Input: part model. Units: mm. Frame: model coordinates. Face numbers are marked on the shaded views. A direction names the side the tool comes from. Give positions to 0.01 mm unless a question says otherwise; leave off trailing zeros. Order: outer loops, then holes, each group sorted by start corner. A loop starts at its lowest first (then second) coordinate and runs counter-clockwise, first axis right, second up. Notation, with made-up numbers: (-5, 24) - (8, 24) arc R21 ccw to (8, 29) - close; hole circle Ø3 at (8, 16). An arc over 180 degrees is marked (long way). Answer in a Markdown table with one row per item. Add a question column.
1. Section query C-C on z = 1.75. Return loops of the section in (x, y), and give its area (3 significant figures).
2. Access query for the marked faces 4, 5, 6, 7 and 8. Directions: +Z, -Z, +X, -X, +Y, -Y. A direction counts if a zero-diameter tool reaches every point of the face in a straight line with its end or side. Return the directions, or none.
3. Ray query, line 1 (X direction, y = 27, z = 1.5); line 2 (Y direction, x = -1.5, z = 0); line 3 (Z direction, x = -10.5, y = 8). Return the intervals inside material, ascending. Write a range as [from, to].
4. Section query D-D on x = -16. Return loops of the section in (y, z).
5. Mould query, pull axis X, two halves, no side actions, for the marked faces 1, 2 and 3. Classes: released by +X, released by -X, zero draft, split by the parting line, or undercut.
6. Section query B-B on x = -2.5. Return loops of the section in (y, z), and give its area (3 significant figures).
7. Contact query for flat-ended pins moving along their axis: pin 1 (6.5 mm diameter, centred on y = 19.5, z = 3, fed in from +X); pin 2 (1.5 mm diameter, centred on x = 7.5, y = 13, fed in from +Z); pin 3 (4 mm diameter, centred on x = -6.5, y = 9, fed in from -Z). Output: stop coordinate, or through.
8. Section query A-A on y = 17.5. Return loops of the section in (x, z).
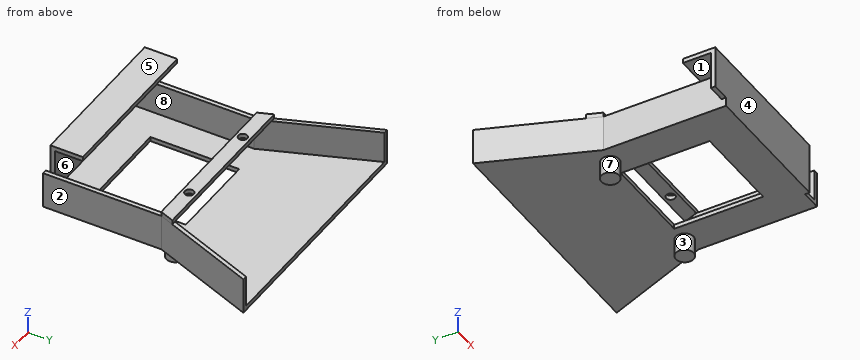
```python
from build123d import *

# Parameters (mm, degrees)
F0_W      = 16.1925
F0_H      = 15.875
F1_DEPTH  = 0.3175
F3_DEPTH  = 5.715
F5_DEPTH  = 0.79375
F6_R      = 0.79375
F7_DEPTH  = 0.79375
F8_DEPTH  = 0.3175
F9_W      = 1.5875
F9_H      = 0.635
F10_DEPTH = 1.5875
F11_DEPTH = 0.3175
F12_W     = 1.5875
F12_H     = 1.5875
F13_DEPTH = 0.79375
F14_DEPTH = 0.15875
F15_R     = 0.5
F16_DEPTH = 25.4
F17_R     = 1.5875
F18_DEPTH = 3.175
F19_DEPTH = 1.5875
F20_DEPTH = 12.7
F21_R     = 0.5
F22_DEPTH = 25.30475
F23_W     = 1.5875
F23_H     = 1.5875
F24_DEPTH = 3.27025
F25_W     = 28.575
F25_H     = 0.79375
F26_DEPTH = 7.62
F27_DEPTH = 0.79375
F28_DEPTH = 0.79375
F29_DEPTH = 0.79375
F30_DEPTH = 25.4
F31_W     = 28.575
F31_H     = 0.79375
F32_DEPTH = 4.998339


with BuildPart() as f1:
    # F0 (on Top) → F1 (new body)
    with BuildSketch(Plane.XY):
        Polygon((-25.671613648, 46.3675076752), (-18.369113648, 27.4050211887), (-18.369113648, 7.0850211887), (10.523386352, 7.0850211887), (10.523386352, 27.4050211887), (17.825886352, 46.3675076752), align=None)
        with Locations((-3.922863648, 20.1025211887)):
            Rectangle(F0_W, F0_H, mode=Mode.SUBTRACT)
    extrude(amount=F1_DEPTH)

    # F2 (on face) → F3 (join)
    with BuildSketch(Plane.XY.offset(0.3175)):
        Polygon((17.825886352, 46.3675076752), (17.032136352, 46.3675076752), (9.729636352, 27.4050211887), (9.729636352, 7.0850211887), (10.523386352, 7.0850211887), (10.523386352, 27.4050211887), align=None)
        Polygon((-24.877863648, 46.3675076752), (-25.671613648, 46.3675076752), (-18.369113648, 27.4050211887), (-18.369113648, 7.0850211887), (-17.575363648, 7.0850211887), (-17.575363648, 27.4050211887), align=None)
    extrude(amount=F3_DEPTH)

    # F4 (on face) → F5 (join)
    with BuildSketch(Plane.XY.offset(6.0325)):
        Polygon((-19.3472738705, 29.9450211887), (-18.369113648, 27.4050211887), (10.523386352, 27.4050211887), (11.5015465745, 29.9450211887), align=None)
    extrude(amount=F5_DEPTH)

    # F6 (on face) → F7 (cut)
    with BuildSketch(Plane.XY.offset(6.82625)):
        with Locations((-12.019113648, 28.6750211887)):
            Circle(F6_R)
        with Locations((4.173386352, 28.6750211887)):
            Circle(F6_R)
    extrude(amount=-F7_DEPTH, mode=Mode.SUBTRACT)

    # F8 (add): a face of the model
    f8_faces = [f1.faces().sort_by_distance(p)[0] for p in [
        (-3.922863648, 30.216271867, 0),
    ]]
    extrude(f8_faces, amount=F8_DEPTH)

    # F9 (on face) → F10 (join)
    with BuildSketch(Plane.XZ.offset(-7.0850211887)):
        Polygon((-17.575363648, 0.3175), (-18.369113648, 0.3175), (-18.369113648, -0.3175), (-16.781613648, -0.3175), (-16.781613648, 0.3175), align=None)
        with Locations((-14.400363648, 0)):
            Rectangle(F9_W, F9_H)
        with Locations((1.379386352, 0)):
            Rectangle(F9_W, F9_H)
        with Locations((4.554386352, 0)):
            Rectangle(F9_W, F9_H)
    extrude(amount=F10_DEPTH)

    # F11 (add): a face of the model
    f11_faces = [f1.faces().sort_by_distance(p)[0] for p in [
        (-3.9482759262, 29.9813117116, -0.3175),
    ]]
    extrude(f11_faces, amount=F11_DEPTH)

    # F12 (on face) → F13 (join)
    with BuildSketch(Plane.XY.offset(0.3175)):
        with Locations((-17.575363648, 6.2912711887)):
            Rectangle(F12_W, F12_H)
        with Locations((-14.400363648, 6.2912711887)):
            Rectangle(F12_W, F12_H)
        with Locations((1.379386352, 6.2912711887)):
            Rectangle(F12_W, F12_H)
        with Locations((4.554386352, 6.2912711887)):
            Rectangle(F12_W, F12_H)
    extrude(amount=F13_DEPTH)

    # F14 (cut): a face of the model
    f14_faces = [f1.faces().sort_by_distance(p)[0] for p in [
        (-3.9482759262, 29.9813117116, -0.635),
    ]]
    extrude(f14_faces, amount=-F14_DEPTH, mode=Mode.SUBTRACT)

    # F15 (on face) → F16 (cut)
    with BuildSketch(Plane(origin=(-18.369113648, 0, 0), x_dir=(0, -1, 0), z_dir=(-1, 0, 0))):
        with Locations((-6.2912711887, 0.3175)):
            Circle(F15_R)
    extrude(amount=-F16_DEPTH, mode=Mode.SUBTRACT)

    # F17 (on face) → F18 (join)
    with BuildSketch(Plane(origin=(0, 0, -0.47625), x_dir=(1, 0, 0), z_dir=(0, 0, -1))):
        with Locations((-15.194113648, -28.0400211887)):
            Circle(F17_R)
        with Locations((7.348386352, -28.0400211887)):
            Circle(F17_R)
    extrude(amount=F18_DEPTH)

    # F19 (add): faces of the model
    f19_faces = [f1.faces().sort_by_distance(p)[0] for p in [
        (5.348136352, 7.0625705484, -0.079375),
        (2.173136352, 7.0625705484, -0.079375),
        (-16.781613648, 7.0625705484, -0.079375),
        (-13.606613648, 7.0625705484, -0.079375),
    ]]
    extrude(f19_faces, amount=F19_DEPTH)

    # F20 (add): a face of the model
    f20_faces = [f1.faces().sort_by_distance(p)[0] for p in [
        (-12.019113648, 6.2912711887, -0.4537993597),
    ]]
    extrude(f20_faces, amount=F20_DEPTH)

    # F21 (on face) → F22 (join)
    with BuildSketch(Plane.YZ.offset(6.935636352)):
        with Locations((6.2912711887, 0.3175)):
            Circle(F21_R)
    extrude(amount=-F22_DEPTH)

    # F23 (on face) → F24 (join)
    with BuildSketch(Plane(origin=(-18.369113648, 0, 0), x_dir=(0, -1, 0), z_dir=(-1, 0, 0))):
        with Locations((-6.2912711887, 0.3175)):
            Rectangle(F23_W, F23_H)
    extrude(amount=F24_DEPTH)

    # F25 (on face) → F26 (join)
    with BuildSketch(Plane.XY.offset(1.11125)):
        with Locations((-7.351863648, 5.8943961887)):
            Rectangle(F25_W, F25_H)
    extrude(amount=F26_DEPTH)

    # F27 (cut): a face of the model
    f27_faces = [f1.faces().sort_by_distance(p)[0] for p in [
        (-5.319863648, 7.0850211887, 0.714375),
    ]]
    extrude(f27_faces, amount=-F27_DEPTH, mode=Mode.SUBTRACT)

    # F28 (add): a face of the model
    f28_faces = [f1.faces().sort_by_distance(p)[0] for p in [
        (-17.972238648, 7.0850211887, 3.571875),
    ]]
    extrude(f28_faces, amount=F28_DEPTH)

    # F29 (add): a face of the model
    f29_faces = [f1.faces().sort_by_distance(p)[0] for p in [
        (8.729511352, 7.0850211887, -0.4019292246),
    ]]
    extrude(f29_faces, amount=F29_DEPTH)

    # F30 (cut): a face of the model
    f30_faces = [f1.faces().sort_by_distance(p)[0] for p in [
        (-20.004238648, 7.0850211887, 0.3175),
    ]]
    extrude(f30_faces, amount=-F30_DEPTH, mode=Mode.SUBTRACT)

    # F31 (on face) → F32 (join)
    with BuildSketch(Plane(origin=(0, 6.2912711887, 0), x_dir=(-1, 0, 0), z_dir=(0, 1, 0))):
        with Locations((7.351863648, 8.334375)):
            Rectangle(F31_W, F31_H)
    extrude(amount=F32_DEPTH)


solid = f1.part
```
Answer:
| question | item | result |
|---|---|---|
| 1 | outline | (-25.67, 46.37) - (-18.37, 27.41) - (-18.37, 6.29) - (-21.64, 6.29) - (-21.64, 5.5) - (6.94, 5.5) - (6.94, 6.29) - (-17.58, 6.29) - (-17.58, 27.41) - (-24.88, 46.37) - close; (9.73, 6.29) - (10.52, 6.29) - (10.52, 27.41) - (17.83, 46.37) - (17.03, 46.37) - (9.73, 27.41) - close |
| 1 | area | 86.3 mm² |
| 2 | face 4 | +Z, -Z, +X, -X, -Y |
| 2 | face 5 | +Z, +X, -X, +Y, -Y |
| 2 | face 6 | none |
| 2 | face 7 | -Z |
| 2 | face 8 | +Y |
| 3 | line 1 | x = [-18.37, -17.58], [9.73, 10.52] |
| 3 | line 2 | y = [5.5, 12.17], [28.04, 46.37] |
| 3 | line 3 | z = [-0.48, 0.32], [7.94, 8.73] |
| 4 | outline | (5.5, -0.48) - (26.67, -0.48) - (26.67, -3.65) - (29.41, -3.65) - (29.41, -0.48) - (46.37, -0.48) - (46.37, 0.32) - (6.29, 0.32) - (6.29, 7.94) - (11.29, 7.94) - (11.29, 8.73) - (5.5, 8.73) - close; (27.41, 6.03) - (29.95, 6.03) - (29.95, 6.83) - (27.41, 6.83) - close |
| 5 | face 1 | zero draft |
| 5 | face 2 | released by +X |
| 5 | face 3 | undercut |
| 6 | outline | (5.5, -0.48) - (12.17, -0.48) - (12.17, 0.32) - (6.29, 0.32) - (6.29, 7.94) - (11.29, 7.94) - (11.29, 8.73) - (5.5, 8.73) - close; (27.41, 6.03) - (29.95, 6.03) - (29.95, 6.83) - (27.41, 6.83) - close; (28.04, -0.48) - (46.37, -0.48) - (46.37, 0.32) - (28.04, 0.32) - close |
| 6 | area | 32.5 mm² |
| 7 | pin 1 | stops at x = 10.52 |
| 7 | pin 2 | stops at z = 0.32 |
| 7 | pin 3 | stops at z = -0.48 |
| 8 | outline | (-18.37, -0.48) - (-12.02, -0.48) - (-12.02, 0.32) - (-17.58, 0.32) - (-17.58, 6.03) - (-18.37, 6.03) - close; (4.17, -0.48) - (10.52, -0.48) - (10.52, 6.03) - (9.73, 6.03) - (9.73, 0.32) - (4.17, 0.32) - close |
